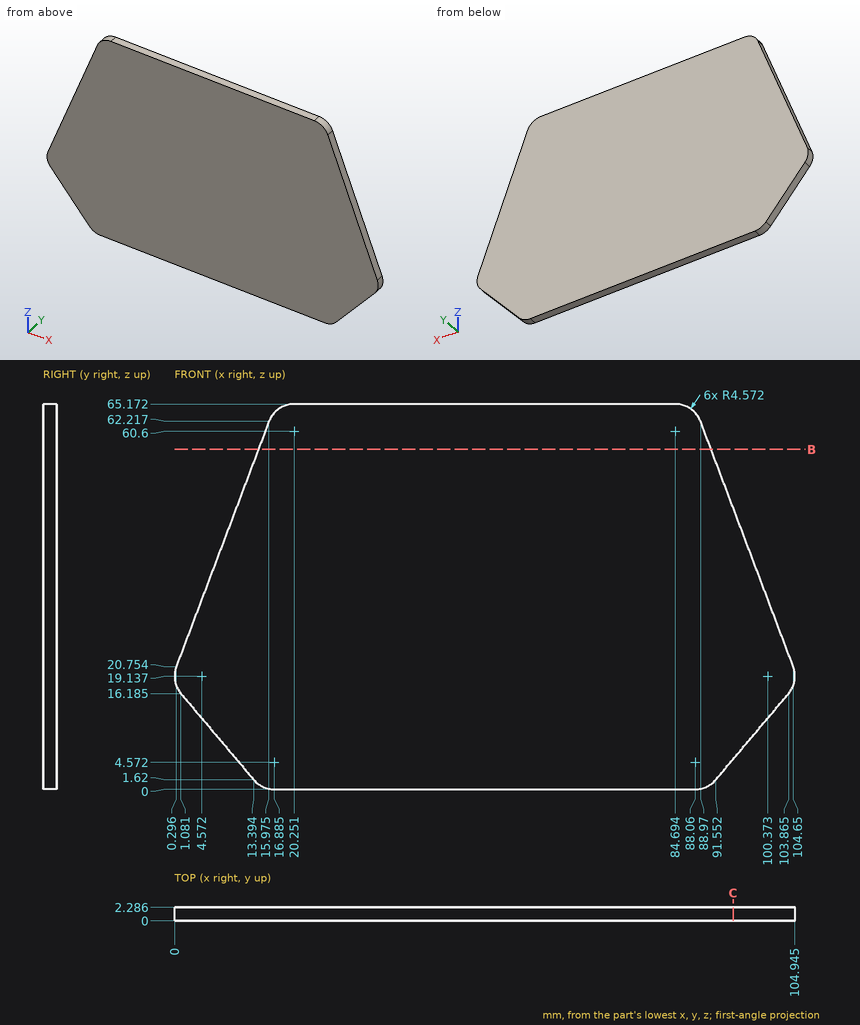
Job drawing, mm, ordinate dimensions from the low corner. One solid piece. Give positions to 0.01 mm unless a question says otherwise; leave off trailing zeros. Order: outer loops, then holes, each group sorted by start corner. A loop starts at its lowest first (then second) coordinate and runs counter-clockwise, first axis right, second up. Notation, with made-up numbers: (-21.75, 81) - (-12.75, 81) arc R19 ccw to (-12.75, 103) - close; hole circle Ø4 at (44, 44). An arc over 180 degrees is marked (long way). One line per question, with ' | ' between items.
1. Drill centre lines: probe 1 along X at (y, z) = (0.2, 3) (1 decimal); probe 2 along X at (y, z) = (0.4, 25) (1 decimal). Where is each one in solid material? Low to high.
Filled in:
probe 1: 12.2 to 92.7 | probe 2: 1.9 to 103
2. Band-saw the part on C-C on x = 94.5. List the corners of the cut face in (y, z) (1 decimal).
Filled in:
outline: (0, 5.1) - (2.3, 5.1) - (2.3, 47.6) - (0, 47.6) - close
3. Band-saw the part on B-B on z = 57.5. List the corners of the cut face in (x, y) (1 decimal).
Filled in:
outline: (14.2, 0) - (90.8, 0) - (90.8, 2.3) - (14.2, 2.3) - close
4. Drop a flat-ended pin along its axis: P1, Ø12, axis at x = 14, z = 21.5, coming from the -Y side. Give the stop position or say it passes through.
Filled in:
P1: y = 0
